Geometry check sheet. Reference: the model listing, model coordinates, mm. A direction names the side the tool comes from. Coordinates: 2 decimals unless noted, no trailing zeros. Loops run counter-clockwise (first coordinate to the right, second up) from the corner with the lowest first, then second, coordinate; pieces in that order, holes last. Notation, with made-up numbers: (28.25, -40) - (85.25, -40) arc R26 cw to (85.25, -18) - close; hole circle Ø2 at (2.5, 23). An arc over 180 degrees is marked (long way). Write each question's results on one line, items separated by ' | '. Start each with the question number.
(1) Material ranges on probe 1 along X at (y, z) = (-22, 34); probe 2 along Y at (x, z) = (-40, 3) (3 decimals); probe 3 along X at (y, z) = (107, 36), recorded low to high.
(2) Sectioned sample at A-A (z = 112.5). Enter the section's corners in (x, y), plus the area to 3 significant figures.
(3) Mould release check, pull along Y, two halves, no side actions. Record for faces 1 (the face through (-3.32, -27, 70)), 2 (the face through (-108.73, 20, 5)): pulls with the +Y half, pulls with the -Y half, needs draft (parallel to the pull), parting line crosses it, or undercut.
(4) Access from +Z, -Z, +X, -X, +Y, -Y to the whole of each face (thin tool, end or side, straight path). Record for faces 3 (the face through (-57, -68.73, 97)), 4 (the face through (22.37, -72, 84)), 5 (the face through (48.293, -67.323, 4.93)).
(5) Sectioned sample at B-B (y = 44.5). Enter the section's corners in (x, z), plus the area to 3 significant figures.
(6) Go/stop test with flat-tipped pins: pin 1 Ø3 at (x, y) = (-59.5, -69.5) entering from -Z; pin 2 Ø10 at (x, z) = (41, 49) entering from +Y; pin 3 Ø2 at (x, z) = (-43.5, 16) entering from +Y. Record where each tip stops, or that it passes through.
(7) Sectioned sample at C-C (x = -40). State how many separate pieces and enclosed holes the cut face has, plus the area to 3 significant figures.
from build123d import *

# Parameters (mm, degrees)
SKETCH1_W            = 230.16
SKETCH1_H            = 130.080000074
BOSS_EXTRUDE1_DEPTH  = 15
SKETCH2_R            = 3.175
CUT_EXTRUDE1_DEPTH   = 10
BOSS_EXTRUDE2_DEPTH  = 230.16
SKETCH5_W            = 6.35
SKETCH5_H            = 130.080000074
SKETCH5_W_2          = 6.64
BOSS_EXTRUDE3_DEPTH  = 127
SKETCH6_W            = 55.554601445
SKETCH6_H            = 12.7
SKETCH6_W_2          = 55.555398555
BOSS_EXTRUDE4_DEPTH  = 57.15
SKETCH17_W           = 6.35
SKETCH17_H           = 57.15
BOSS_EXTRUDE9_DEPTH  = 76.2
SKETCH18_W           = 15.24
SKETCH18_H           = 31.75
CUT_EXTRUDE2_DEPTH   = 69.85
SKETCH19_W           = 3.81
SKETCH19_H           = 31.75
SKETCH19_W_2         = 4.79
BOSS_EXTRUDE10_DEPTH = 25.4
SKETCH20_W           = 230.16
SKETCH20_H           = 61.2
BOSS_EXTRUDE12_DEPTH = 6.35
SKETCH21_R           = 1.190625
SKETCH21_W           = 12.7
SKETCH21_H           = 23.8125
CUT_EXTRUDE3_DEPTH   = 6.35


with BuildPart() as part:
    # Sketch1 → Boss-Extrude1 (new body)
    with BuildSketch(Plane.XY):
        with Locations((0, -10.039999963)):
            Rectangle(SKETCH1_W, SKETCH1_H)
    extrude(amount=BOSS_EXTRUDE1_DEPTH)

    # Sketch2 → Cut-Extrude1 (cut)
    with BuildSketch(Plane(origin=(0, 0, 0), x_dir=(-1, 0, 0), z_dir=(0, 0, -1))):
        with Locations((60, -70)):
            Circle(SKETCH2_R)
        with Locations((50, -70)):
            Circle(SKETCH2_R)
        with Locations((40, -70)):
            Circle(SKETCH2_R)
        with Locations((-40, -70)):
            Circle(SKETCH2_R)
        with Locations((-50, -70)):
            Circle(SKETCH2_R)
        with Locations((-60, -70)):
            Circle(SKETCH2_R)
        with Locations((-110, 10)):
            Circle(SKETCH2_R)
        with Locations((-110, 20)):
            Circle(SKETCH2_R)
        with Locations((-110, 30)):
            Circle(SKETCH2_R)
        with Locations((110, 10)):
            Circle(SKETCH2_R)
        with Locations((110, 20)):
            Circle(SKETCH2_R)
        with Locations((110, 30)):
            Circle(SKETCH2_R)
    extrude(amount=-CUT_EXTRUDE1_DEPTH, mode=Mode.SUBTRACT)

    # Sketch4 → Boss-Extrude2 (add)
    with BuildSketch(Plane.ZY.offset(115.08)):
        Polygon((15, -75.08), (15, 55.000000074), (40.4, 55.000000074), align=None)
    extrude(amount=-BOSS_EXTRUDE2_DEPTH)

    # Sketch5 → Boss-Extrude3 (add)
    with BuildSketch(Plane(origin=(0, 0, 0), x_dir=(-1, 0, 0), z_dir=(0, 0, -1))):
        with Locations((111.905, -10.039999963)):
            Rectangle(SKETCH5_W, SKETCH5_H)
        with Locations((-111.905, -10.039999963)):
            Rectangle(SKETCH5_W, SKETCH5_H)
        with Locations((0, -10.039999963)):
            Rectangle(SKETCH5_W_2, SKETCH5_H)
    extrude(amount=-BOSS_EXTRUDE3_DEPTH)

    # Sketch6 → Boss-Extrude4 (add)
    with BuildSketch(Plane(origin=(0, 55.000000074, 0), x_dir=(1, 0, 0), z_dir=(0, 1, 0))):
        with Locations((-80.952699278, -34.05)):
            Rectangle(SKETCH6_W, SKETCH6_H)
        with Locations((80.952300722, -34.05)):
            Rectangle(SKETCH6_W_2, SKETCH6_H)
    extrude(amount=BOSS_EXTRUDE4_DEPTH)

    # Sketch14 → Loft1 section 0
    with BuildSketch(Plane.ZY.offset(108.73)):
        with BuildLine():
            Line((40.4, 67.540000074), (40.4, 112.150000074))
            Line((40.4, 112.150000074), (46.75, 112.150000074))
            Line((46.75, 112.150000074), (40.4, 67.540000074))
        make_face()
    # Sketch13 → Loft1 section 1
    with BuildSketch(Plane(origin=(-15.075398555, 0, 0), x_dir=(0, 0, -1), z_dir=(1, 0, 0))):
        with BuildLine():
            Line((-40.4, 112.150000074), (-40.4, 67.540000074))
            Line((-40.4, 67.540000074), (-53.1, 112.150000074))
            Line((-53.1, 112.150000074), (-40.4, 112.150000074))
        make_face()
    loft()

    # Sketch15 → Loft2 section 0
    with BuildSketch(Plane.ZY.offset(-15.074601445)):
        with BuildLine():
            Line((53.1, 112.150000074), (40.4, 67.540000074))
            Line((40.4, 67.540000074), (40.4, 112.150000074))
            Line((40.4, 112.150000074), (53.1, 112.150000074))
        make_face()
    # Sketch16 → Loft2 section 1
    with BuildSketch(Plane(origin=(108.73, 0, 0), x_dir=(0, 0, -1), z_dir=(1, 0, 0))):
        with BuildLine():
            Line((-40.4, 112.150000074), (-46.75, 112.150000074))
            Line((-46.75, 112.150000074), (-40.4, 67.540000074))
            Line((-40.4, 67.540000074), (-40.4, 112.150000074))
        make_face()
    loft()

    # Sketch17 → Boss-Extrude9 (add)
    with BuildSketch(Plane(origin=(0, 0, 27.7), x_dir=(-1, 0, 0), z_dir=(0, 0, -1))):
        Polygon((-115.08, 112.150000074), (-108.73, 112.150000074), (-53.174601445, 112.150000074), (-53.174601445, 118.500000074), (-115.08, 118.500000074), align=None)
        with Locations((-111.905, 83.575000074)):
            Rectangle(SKETCH17_W, SKETCH17_H)
        Polygon((108.73, 112.150000074), (115.08, 112.150000074), (115.08, 118.500000074), (53.175398555, 118.500000074), (53.175398555, 112.150000074), align=None)
        with Locations((111.905, 83.575000074)):
            Rectangle(SKETCH17_W, SKETCH17_H)
    extrude(amount=-BOSS_EXTRUDE9_DEPTH)

    # Sketch18 → Cut-Extrude2 (cut)
    with BuildSketch(Plane.XY.offset(127)):
        with Locations((-0.33125, 39.125000074)):
            Rectangle(SKETCH18_W, SKETCH18_H)
    extrude(amount=-CUT_EXTRUDE2_DEPTH, mode=Mode.SUBTRACT)

    # Sketch19 → Boss-Extrude10 (add)
    with BuildSketch(Plane.XY.offset(57.15)):
        with Locations((5.225, 39.125000074)):
            Rectangle(SKETCH19_W, SKETCH19_H)
        with Locations((-5.715, 39.125000074)):
            Rectangle(SKETCH19_W_2, SKETCH19_H)
    extrude(amount=-BOSS_EXTRUDE10_DEPTH)

    # Sketch20 → Boss-Extrude12 (add)
    with BuildSketch(Plane.XZ.offset(75.08)):
        with Locations((0, 96.4)):
            Rectangle(SKETCH20_W, SKETCH20_H)
    extrude(amount=-BOSS_EXTRUDE12_DEPTH)

    # Sketch21 → Cut-Extrude3 (cut)
    with BuildSketch(Plane.XZ.offset(75.08)):
        with Locations(Location((-16.02, 69.76875, 0), (0, 0, 270))):
            Circle(SKETCH21_R)
        with Locations(Location((-16.02, 98.34375, 0), (0, 0, 270))):
            Circle(SKETCH21_R)
        with Locations(Location((16.02, 69.76875, 0), (0, 0, 270))):
            Circle(SKETCH21_R)
        with Locations(Location((16.02, 98.34375, 0), (0, 0, 270))):
            Circle(SKETCH21_R)
        with Locations((-16.02, 84.05625)):
            Rectangle(SKETCH21_W, SKETCH21_H)
        with Locations((16.02, 84.05625)):
            Rectangle(SKETCH21_W, SKETCH21_H)
    extrude(amount=-CUT_EXTRUDE3_DEPTH, mode=Mode.SUBTRACT)


solid = part.part
Outcome:
1) probe 1: x = -115.08 to -108.73, -3.32 to 3.32, 108.73 to 115.08 | probe 2: y = -75.08 to -73.175, -66.825 to 55 | probe 3: x = -115.08 to -53.18, 53.17 to 115.08
2) outline: (-115.08, -75.08) - (115.08, -75.08) - (115.08, 55) - (108.73, 55) - (108.73, -68.73) - (3.32, -68.73) - (3.32, 23.25) - (-3.32, 23.25) - (-3.32, -68.73) - (-108.73, -68.73) - (-108.73, 55) - (-115.08, 55) - close | area: 3,640 mm2
3) face 1: needs draft | face 2: undercut
4) face 3: +Z | face 4: +Y, -Y | face 5: -Z
5) outline: (-115.08, 0) - (115.08, 0) - (115.08, 127) - (108.73, 127) - (108.73, 38.35) - (7.13, 38.35) - (7.13, 57.15) - (-8.11, 57.15) - (-8.11, 38.35) - (-108.73, 38.35) - (-108.73, 127) - (-115.08, 127) - close | area: 10,200 mm2
6) pin 1: stops at z = 10 | pin 2: stops at y = 112.15 | pin 3: stops at y = 55
7) separate pieces: 3 | enclosed holes: 0 | area: 4,170 mm2
